```python
from build123d import *

# Parameters (mm, degrees)
SKETCH1_W               = 90
SKETCH1_H               = 12
BOSS_EXTRUDE1_DEPTH     = 2
SKETCH2_W               = 90
SKETCH2_H               = 2
BOSS_EXTRUDE2_DEPTH     = 10
CUT_EXTRUDE1_DEPTH      = 63.420894383
CUT_EXTRUDE1_DEPTH_BACK = 63.420894383
SKETCH3_R               = 2.5
CUT_EXTRUDE2_DEPTH      = 64.477248768
CUT_EXTRUDE2_DEPTH_BACK = 64.477248768
SKETCH4_R               = 2.5


with BuildPart() as part:
    # Sketch1 → Boss-Extrude1 (new body)
    with BuildSketch(Plane(origin=(0, 0, 0), x_dir=(1, 0, 0), z_dir=(0, 1, 0))):
        with Locations((-16.166666667, 1.416666667)):
            Rectangle(SKETCH1_W, SKETCH1_H)
    extrude(amount=BOSS_EXTRUDE1_DEPTH)

    # Sketch2 → Boss-Extrude2 (add)
    with BuildSketch(Plane(origin=(0, 2, 0), x_dir=(1, 0, 0), z_dir=(0, 1, 0))):
        with Locations((-16.166666667, 6.416666667)):
            Rectangle(SKETCH2_W, SKETCH2_H)
    extrude(amount=BOSS_EXTRUDE2_DEPTH)

    # Sketch3 → Cut-Extrude1 (cut, two sides: drawn at the far end of the back side and taken through both)
    with BuildSketch(Plane(origin=(0, 2, 0), x_dir=(1, 0, 0), z_dir=(0, 1, 0)).offset(-CUT_EXTRUDE1_DEPTH_BACK)):
        with Locations(Location((-28.666666667, 0.416666667, 0), (0, 0, 270))):
            Circle(SKETCH3_R)
        with Locations(Location((-3.666666667, 0.416666667, 0), (0, 0, 270))):
            Circle(SKETCH3_R)
    extrude(amount=CUT_EXTRUDE1_DEPTH + CUT_EXTRUDE1_DEPTH_BACK, mode=Mode.SUBTRACT)

    # Sketch4 → Cut-Extrude2 (cut, two sides: drawn at the far end of the back side and taken through both)
    with BuildSketch(Plane(origin=(0, 0, -7.416666667), x_dir=(-1, 0, 0), z_dir=(0, 0, -1)).offset(-CUT_EXTRUDE2_DEPTH_BACK)):
        with Locations((-13.833333333, 7)):
            Circle(SKETCH4_R)
        with Locations((16.166666667, 7)):
            Circle(SKETCH4_R)
        with Locations((46.166666667, 7)):
            Circle(SKETCH4_R)
    extrude(amount=CUT_EXTRUDE2_DEPTH + CUT_EXTRUDE2_DEPTH_BACK, mode=Mode.SUBTRACT)


solid = part.part
```
Read the model definition and answer for the solid it produces. Units are mm, in the model's axes. A direction names the side the tool comes from. Coordinates: 2 decimals unless noted, no trailing zeros. Loops run counter-clockwise (first coordinate to the right, second up) from the corner with the lowest first, then second, coordinate; pieces in that order, holes last. Notation, with made-up numbers: (-16.75, 72) - (19.25, 72) arc R19 cw to (19.25, 107) - close; hole circle Ø2 at (73, 76). An arc over 180 degrees is marked (long way). Answer in a Markdown table with one row per item.
1. Straight lines are drawn through the part: line 1 (X direction, y = 7, z = -5.9); line 2 (X direction, y = 6, z = -6); line 3 (Y direction, x = -46, z = -2.25). For each, find the intervals that lie inside material, in ascending order.
Conclusion:
| item | result |
|---|---|
| line 1 | x = -61.17 to -48.67, -43.67 to -18.67, -13.67 to 11.33, 16.33 to 28.83 |
| line 2 | x = -61.17 to -48.46, -43.88 to -18.46, -13.88 to 11.54, 16.12 to 28.83 |
| line 3 | y = 0 to 2 |
2. Find section C-C, the plane x = 21. Write down the section's boundary in (y, z).
Conclusion:
| item | result |
|---|---|
| outline | (0, -7.42) - (12, -7.42) - (12, -5.42) - (2, -5.42) - (2, 4.58) - (0, 4.58) - close |
3. Find section B-B, the plane z = 0. Write down the section's boundary in (x, y), then the cut area to 3 significant figures.
Conclusion:
| item | result |
|---|---|
| outline | (-61.17, 0) - (-31.13, 0) - (-31.13, 2) - (-61.17, 2) - close; (-26.2, 0) - (-6.13, 0) - (-6.13, 2) - (-26.2, 2) - close; (-1.2, 0) - (28.83, 0) - (28.83, 2) - (-1.2, 2) - close |
| area | 160 mm² |
4. Find section D-D, the plane y = 10.25. Write down the section's boundary in (x, z).
Conclusion:
| item | result |
|---|---|
| outline | (-61.17, -7.42) - (28.83, -7.42) - (28.83, -5.42) - (-61.17, -5.42) - close |
5. Find section A-A, the plane y = 7. Write down the section's boundary in (x, z), then the cut area to 3 significant figures.
Conclusion:
| item | result |
|---|---|
| outline | (-61.17, -7.42) - (-48.67, -7.42) - (-48.67, -5.42) - (-61.17, -5.42) - close; (-43.67, -7.42) - (-18.67, -7.42) - (-18.67, -5.42) - (-43.67, -5.42) - close; (-13.67, -7.42) - (11.33, -7.42) - (11.33, -5.42) - (-13.67, -5.42) - close; (16.33, -7.42) - (28.83, -7.42) - (28.83, -5.42) - (16.33, -5.42) - close |
| area | 150 mm² |
6. Which of the six approach directions +Z, -Z, +X, -X, +Y, -Y give full straight-line access (tool end or side, diameter ignored) to faces 1 (the face through (-17, 4, -5.417)), 2 (the face through (28.833, 1, -3))?
Conclusion:
| item | result |
|---|---|
| face 1 | +Z, +X, -X, +Y |
| face 2 | +Z, -Z, +X, +Y, -Y |
7. Determine the mould class of faces 3 (the face through (-3.557, 0.986, -2.914)), 4 (the face through (-17, 3, -7.417)), 5 (the face through (-18.476, 6.042, -6.403)) for opening direction Z: +Z half, -Z half, draft (parallel to the pull), parting line (faces both ways), or undercut.
Conclusion:
| item | result |
|---|---|
| face 3 | undercut |
| face 4 | -Z half |
| face 5 | draft |
8. Given pin 1 (3 mm diameter, centred on x = -28.67, z = -0.42, fed in from -Y); pin 2 (6.5 mm diameter, centred on x = -16.17, y = 7, fed in from +Z), each flat-ended and moving along its own axis, determine where each tip first touches the part or whether it passes through.
Conclusion:
| item | result |
|---|---|
| pin 1 | passes through |
| pin 2 | stops at z = -5.42 |
